```python
from build123d import *

# Parameters (mm, degrees)
SKETCH1_W           = 250
SKETCH1_H           = 250
BOSS_EXTRUDE1_DEPTH = 3
SKETCH4_R           = 2
CUT_EXTRUDE1_DEPTH  = 3
CUT_EXTRUDE2_DEPTH  = 3


with BuildPart() as part:
    # Sketch1 → Boss-Extrude1 (new body)
    with BuildSketch(Plane(origin=(0, 0, 0), x_dir=(1, 0, 0), z_dir=(0, 1, 0))):
        Rectangle(SKETCH1_W, SKETCH1_H)
    extrude(amount=BOSS_EXTRUDE1_DEPTH)

    # Sketch4 → Cut-Extrude1 (cut)
    with BuildSketch(Plane(origin=(0, 3, 0), x_dir=(1, 0, 0), z_dir=(0, 1, 0))):
        with Locations(Location((91, -28, 0), (0, 0, 270))):
            Circle(SKETCH4_R)
        with Locations(Location((91, -7, 0), (0, 0, 270))):
            Circle(SKETCH4_R)
        with Locations(Location((119, -7, 0), (0, 0, 270))):
            Circle(SKETCH4_R)
        with Locations(Location((119, -28, 0), (0, 0, 270))):
            Circle(SKETCH4_R)
        with Locations(Location((22.62859709, -29, 0), (0, 0, 270))):
            Circle(SKETCH4_R)
        with Locations(Location((22.62859709, 33, 0), (0, 0, 270))):
            Circle(SKETCH4_R)
        with Locations(Location((-73.776388534, 25, 0), (0, 0, 270))):
            Circle(SKETCH4_R)
        with Locations(Location((-73.776388534, -21, 0), (0, 0, 270))):
            Circle(SKETCH4_R)
        with Locations(Location((-91, -28, 0), (0, 0, 270))):
            Circle(SKETCH4_R)
        with Locations(Location((-91, -7, 0), (0, 0, 270))):
            Circle(SKETCH4_R)
        with Locations(Location((-119, -7, 0), (0, 0, 270))):
            Circle(SKETCH4_R)
        with Locations(Location((-119, -28, 0), (0, 0, 270))):
            Circle(SKETCH4_R)
    extrude(amount=-CUT_EXTRUDE1_DEPTH, mode=Mode.SUBTRACT)

    # Sketch5 → Cut-Extrude2 (cut)
    with BuildSketch(Plane(origin=(0, 3, 0), x_dir=(1, 0, 0), z_dir=(0, 1, 0))):
        Polygon((2.62859709, -110), (-60, -110), (-60, -84), (-64, -84), (-64, 80), (2.62859709, 80), align=None)
        Polygon((37.62859709, 80), (37.62859709, -110), (60, -110), (60, -84), (76, -84), (76, 80), align=None)
    extrude(amount=-CUT_EXTRUDE2_DEPTH, mode=Mode.SUBTRACT)


solid = part.part
```
Verification items for the finished model (mm, model axes). Coordinates: 2 decimals unless noted, no trailing zeros. Loops run counter-clockwise (first coordinate to the right, second up) from the corner with the lowest first, then second, coordinate; pieces in that order, holes last. Notation, with made-up numbers: (7.5, -8.75) - (26.5, -8.75) arc R12 ccw to (26.5, 7.25) - close; hole circle Ø5 at (61, 7.5). An arc over 180 degrees is marked (long way). Answer as a JSON object with one key per item and string values.
(1) Cross-section at B-B, the plane y = 2.1. Count the separate pieces of the cut face and the enclosed holes in it, then the cut area to 3 significant figures.
Response:
{"separate pieces": "1", "enclosed holes": "14", "area": "42,900 mm²"}
(2) Go/stop test with a flat-tipped pin: pin 1 Ø5 at (x, z) = (22.63, 29) entering from -Y. Record where the tip stops, or that it passes through.
Response:
{"pin 1": "stops at y = 0"}
(3) Scan lines: line 1 along X through (y, z) = (0.5, 32); line 2 along X through (y, z) = (0.55, 105.5); line 3 along X through (y, z) = (0.9, -33). Record each from-to range of solid material in increasing order.
Response:
{"line 1": "x = -125 to -64, 2.63 to 37.63, 76 to 125", "line 2": "x = -125 to -60, 2.63 to 37.63, 60 to 125", "line 3": "x = -125 to -64, 2.63 to 20.63, 24.63 to 37.63, 76 to 125"}
(4) Cross-section at A-A, the plane z = -74. Record the boundary of the cut face in (x, y).
Response:
{"outline": "(-125, 0) - (-64, 0) - (-64, 3) - (-125, 3) - close; (2.63, 0) - (37.63, 0) - (37.63, 3) - (2.63, 3) - close; (76, 0) - (125, 0) - (125, 3) - (76, 3) - close"}
(5) Cross-section at C-C, the plane z = 100. Record the boundary of the cut face in (x, y).
Response:
{"outline": "(-125, 0) - (-60, 0) - (-60, 3) - (-125, 3) - close; (2.63, 0) - (37.63, 0) - (37.63, 3) - (2.63, 3) - close; (60, 0) - (125, 0) - (125, 3) - (60, 3) - close"}
